Part model, mm, in its own coordinate system. Round coordinates to 2 decimals unless told otherwise and drop trailing zeros. Order: outer loops, then holes, each group sorted by start corner. A loop starts at its lowest first (then second) coordinate and runs counter-clockwise, first axis right, second up. Notation, with made-up numbers: (-27, 13) -> (-10, 13) arc R36 cw to (-10, 52) -> close; hole circle Ø2 at (-14, 68). An arc over 180 degrees is marked (long way). Return JSON: item names as keys, results as strings. Group by question number.
from build123d import *

# Parameters (mm, degrees)
EXTRUSION1_DEPTH          = 3
ESQUISSE3_R               = 5.5
ENL_V_MAT_EXTRU_1_DEPTH   = 4
CONG_1_R                  = 12
TROU_TARAUD_M5X0_82_D     = 4.2
TROU_TARAUD_M5X0_82_DEPTH = 3
TROU_TARAUD_M5X0_82_TIP   = 1.2618073


with BuildPart() as part:
    # Esquisse2 → Extrusion1 (new body)
    with BuildSketch(Plane.XY):
        Polygon((-5.959878762, 64.527559487), (18.544923687, 66.671451903), (34.040121238, 63.939230504), (34.040121238, -14.560769496), (14.544923687, -16.266378275), (-5.959878762, -14.472440513), align=None)
    extrude(amount=EXTRUSION1_DEPTH)

    # Esquisse3 → Enlèv. mat.-Extru.1 (cut, through all)
    with BuildSketch(Plane.XY.offset(3)):
        with Locations((9.040121238, 37.527559487)):
            Circle(ESQUISSE3_R)
    extrude(amount=-ENL_V_MAT_EXTRU_1_DEPTH, mode=Mode.SUBTRACT)

    # Congé1
    cong_1_edges = [part.edges().sort_by_distance(p)[0] for p in [
        (-5.959878762, 64.527559487, 1.5),
        (-5.959878762, -14.472440513, 1.5),
        (34.040121238, 63.939230504, 1.5),
        (34.040121238, -14.560769496, 1.5),
    ]]
    fillet(cong_1_edges, radius=CONG_1_R)

    # Trou taraudé M5x0.82
    with Locations(Plane(origin=(1.540121238, 54.527559487, 3), x_dir=(1, 0, 0), z_dir=(0, 0, 1))):
        with Locations((0, 0), (16, 2.5), (0, -34), (16, -36.5)):
            Hole(TROU_TARAUD_M5X0_82_D / 2, depth=TROU_TARAUD_M5X0_82_DEPTH)
            with Locations((0, 0, -(TROU_TARAUD_M5X0_82_DEPTH + TROU_TARAUD_M5X0_82_TIP / 2))):  # 118° drill point
                Cone(0, TROU_TARAUD_M5X0_82_D / 2, TROU_TARAUD_M5X0_82_TIP, mode=Mode.SUBTRACT)


solid = part.part
(1) Saw through at C-C, the plane z = 1.35. List the corners of the cut face in (x, y).
(2) Mould opens along X. For faces 1 (the flat face through (14, 26, 3)), 2 (the cylindrical face through (15.6, 17.22, 1.48)), 3 (the cylindrical face through (18, 54.98, 1.48)), 4 (the flat face through (11.67, 66.07, 1.48)) say: pulls with the +X half, pulls with the -X half, needs draft (parallel to the pull), parting line crosses it, or undercut.
(3) Pin check, flat tip, straight feed: P1, Ø6.5, axis at x = 9.04, y = 37.53, coming from the +Z side. Stop position of the tip, or through.
(4) Saw through at B-B, the plane y = 17. List the corners of the cut face in (x, z).
(5) Saw through at D-D, the plane x = -2. List the corners of the cut face in (y, z), and give its area (3 significant figures).
(6) Probe L1, parallel to Y at x = 16, z = 1.6; L2, parallel to Y at x = 19, z = 1.2; L3, parallel to Y at x = 10.5, z = 1.65. List the from-to ranges inside material, lowest first. Write a range as [from, to].
(7) Saw through at A-A, the plane x = 10.5. List the corners of the cut face in (y, z).
Results are:
{
 "1": {"outline": "(-5.96, -3.48) arc R12 ccw to (4.99, -15.43) -> (14.54, -16.27) -> (23.09, -15.52) arc R12 ccw to (34.04, -3.56) -> (34.04, 53.87) arc R12 ccw to (24.12, 65.69) -> (18.54, 66.67) -> (4.99, 65.49) arc R12 ccw to (-5.96, 53.53) -> close; hole circle Ø4.2 at (1.54, 20.53); hole circle Ø4.2 at (1.54, 54.53); hole circle Ø11 at (9.04, 37.53); hole circle Ø4.2 at (17.54, 18.03); hole circle Ø4.2 at (17.54, 57.03)"},
 "2": {"face 1": "needs draft", "face 2": "undercut", "face 3": "undercut", "face 4": "pulls with the -X half"},
 "3": {"P1": "passes through"},
 "4": {"outline": "(-5.96, 0) -> (15.71, 0) -> (15.71, 3) -> (-5.96, 3) -> close; (19.37, 0) -> (34.04, 0) -> (34.04, 3) -> (19.37, 3) -> close"},
 "5": {"outline": "(-12.38, 0) -> (62.44, 0) -> (62.44, 3) -> (-12.38, 3) -> close", "area": "224 mm^2"},
 "6": {"L1": "y = [-16.14, 16.6], [19.46, 55.6], [58.46, 66.45]", "L2": "y = [-15.88, 16.52], [19.54, 55.52], [58.54, 66.59]", "L3": "y = [-15.91, 32.22], [42.83, 65.97]"},
 "7": {"outline": "(-15.91, 0) -> (32.22, 0) -> (32.22, 3) -> (-15.91, 3) -> close; (42.83, 0) -> (65.97, 0) -> (65.97, 3) -> (42.83, 3) -> close"}
}
